The model under review builds one solid part; all positions refer to its coordinate system, in mm. A direction names the side the tool comes from. Round coordinates to 2 decimals unless told otherwise and drop trailing zeros. Order: outer loops, then holes, each group sorted by start corner. A loop starts at its lowest first (then second) coordinate and runs counter-clockwise, first axis right, second up. Notation, with made-up numbers: M 81,87 L 94,87 A20 cw 94,111 Z; hole C 33.25,64.5 d9. An arc over 180 degrees is marked long. One line per item, written item: value. Start each with the question number.
Autodesk Inventor part; units mm, degrees
ref_plane "2_XY" through (0, 3.15, 0) normal (1, 0, 0) x (0, 0, -1)
ref_plane "2_YZ" through (0, 3.15, 0) normal (0, 0, -1) x (0, 1, 0)
ref_plane "2_ZX" through (0, 3.15, 0) normal (0, 1, 0) x (1, 0, 0)
sketch "Sketch_1" plane through (0, 0, 0) normal (0, 1, 0) x (-1, 0, 0)
  line L0 (0, 16) -> (-25, 16)
  line L1 (-25, 16) -> (-25, 3.15)
  line L2 (-25, 3.15) -> (-20, 3.15)
  line L3 (-20, 3.15) -> (-20, 3.65)
  line L4 (-20, 3.65) -> (-15, 3.65)
  line L5 (-15, 3.65) -> (-15, 3.15)
  line L6 (-15, 3.15) -> (-10, 3.15)
  line L7 (-10, 3.15) -> (-10, 3.65)
  line L8 (-10, 3.65) -> (-5, 3.65)
  line L9 (-5, 3.65) -> (-5, 3.15)
  line L10 (-5, 3.15) -> (0, 3.15)
  line L11 (0, 3.15) -> (0, 16)
extrude "Extrusion1" add sketch "Sketch_1" along normal blind 1.5
sketch "Sketch_2" plane through (0, 0, 0) normal (1, 0, 0) x (0, 1, 0)
  line L0 (1.5, 10.6667) -> (0, 10.6667)
  line L1 (0, 10.6667) -> (0, 0)
  arc A0 (0, 0) -> (3.15, 3.15) centre (3.15, 0) ccw
  line L2 (3.15, 3.15) -> (1.5, 3.15)
  line L3 (1.5, 3.15) -> (1.5, 10.6667)
  circle A1 centre (3.15, 0) radius 1.5
extrude "Extrusion2" add sketch "Sketch_2" along normal blind 5
sketch "Sketch_3" plane through (10, 0, 0) normal (1, 0, 0) x (0, 0, -1)
  line L0 (-10.6667, 1.5) -> (-10.6667, 0)
  line L1 (-10.6667, 0) -> (0, 0)
  arc A0 (0, 0) -> (-3.15, 3.15) centre (0, 3.15) ccw
  line L2 (-3.15, 3.15) -> (-3.15, 1.5)
  line L3 (-3.15, 1.5) -> (-10.6667, 1.5)
  circle A1 centre (0, 3.15) radius 1.5
extrude "Extrusion3" add sketch "Sketch_3" along normal blind 5
sketch "Sketch_4" plane through (20, 0, 0) normal (1, 0, 0) x (0, 0, -1)
  line L0 (-10.6667, 1.5) -> (-10.6667, 0)
  line L1 (-10.6667, 0) -> (0, 0)
  arc A0 (0, 0) -> (-3.15, 3.15) centre (0, 3.15) ccw
  line L2 (-3.15, 3.15) -> (-3.15, 1.5)
  line L3 (-3.15, 1.5) -> (-10.6667, 1.5)
  circle A1 centre (0, 3.15) radius 1.5
extrude "Extrusion4" add sketch "Sketch_4" along normal blind 5
sketch "Sketch5" plane through (0, 0, 0) normal (0, -1, 0) x (1, 0, 0)
  point P0 (6, 10)
hole "Hole1" at (6, 0, 10) direction (0, 1, 0) diameter 3.4 depth 2
sketch "Sketch6" plane through (0, 0, 0) normal (0, -1, 0) x (1, 0, 0)
  point P0 (19, 10)
hole "Hole2" at (19, 0, 10) direction (0, 1, 0) diameter 3.4 depth 2
ref_plane "2_XY" through (0, 3.15, 0) normal (1, 0, 0) x (0, 0, -1)
ref_plane "2_YZ" through (0, 3.15, 0) normal (0, 0, -1) x (0, 1, 0)
ref_plane "2_ZX" through (0, 3.15, 0) normal (0, 1, 0) x (1, 0, 0)
properties part number "2HHKS25" material "ステンレス鋼"
Item 1: Consider section A-A, the plane z = 10. Give the boundary of the cut face in (x, y), then the cut area to 3 significant figures.
Item 2: The part is to be moulded in two halves that separate along Z. For faces 4 (the flat face through (22, 2, 3.15)), 5 (the flat face through (10, 1.7, 1)), 6 (the cylindrical face through (2.46, 4.58, -0.45)), say which applies: pulls with the +Z half, pulls with the -Z half, needs draft (parallel to the pull), parting line crosses it, or undercut.
Item 3: Consider section C-C, the plane x = 12. Give the boundary of the cut face in (y, z).
Item 4: Machinability: for faces 1 (the flat face through (2, 2, 3.15)), 2 (the flat face through (5, 1.7, 1.1)), 3 (the cylindrical face through (17.567, 0.76, 9.086)), which of the approach directions +Z, -Z, +X, -X, +Y, -Y give a long, thin tool a straight path to every point of the face, cutting with its end or side? Answer none if there is none.
Item 5: Consider section D-D, the plane y = 3.5. Give the boundary of the cut face in (x, z), then the cut area to 3 significant figures.
Item 6: Consider section B-B, the plane x = 6. Give the boundary of the cut face in (y, z), then the cut area to 3 significant figures.
Item 7: Wall thickness on L1, parallel to X at y = 1, z = -0.75; L2, parallel to X at y = 0.85, z = 10; L3, parallel to Y at x = 12.15, z = 0: over which ranges is each line inside the solid? List them lowest first.
Item 8: Clearance check with flat-ended pins moving along their axes: P1, Ø1.8, axis at x = 21.5, y = 2.5, coming from the +Z side; P2, Ø1.6, axis at x = 16.5, y = 0.5, coming from the -Z side; P3, Ø2, axis at x = 18, z = 3.5, coming from the +Y side; P4, Ø2.5, axis at y = 3.15, z = 0, coming from the -X side. State where each tip first meets the part, or that it passes through.
Computed:
1. outline: M 0,0 L 4.3,0 L 4.3,1.5 L 0,1.5 Z; M 7.7,0 L 17.3,0 L 17.3,1.5 L 7.7,1.5 Z; M 20.7,0 L 25,0 L 25,1.5 L 20.7,1.5 Z
1. area: 27.3 mm^2
2. face 4: pulls with the +Z half
2. face 5: needs draft
2. face 6: undercut
3. outline: M 0,0 A3.15 ccw long 3.15,3.15 L 1.5,3.15 L 1.5,16 L 0,16 Z; hole C 3.15,0 d3
4. face 1: +Z, +X, -X, +Y
4. face 2: -Z, +Y, -Y
4. face 3: +Y, -Y
5. outline: M 0,-3.13 L 5,-3.13 L 5,-1.46 L 0,-1.46 Z; M 0,1.46 L 5,1.46 L 5,3.13 L 0,3.13 Z; M 10,-3.13 L 15,-3.13 L 15,-1.46 L 10,-1.46 Z; M 10,1.46 L 15,1.46 L 15,3.13 L 10,3.13 Z; M 20,-3.13 L 25,-3.13 L 25,-1.46 L 20,-1.46 Z; M 20,1.46 L 25,1.46 L 25,3.13 L 20,3.13 Z
5. area: 50.2 mm^2
6. outline: M 0,3.65 L 1.5,3.65 L 1.5,8.3 L 0,8.3 Z; M 0,11.7 L 1.5,11.7 L 1.5,16 L 0,16 Z
6. area: 13.4 mm^2
7. L1: x = 0 to 5, 10 to 15, 20 to 25
7. L2: x = 0 to 4.3, 7.7 to 17.3, 20.7 to 25
7. L3: y = 0 to 1.65, 4.65 to 6.3
8. P1: stops at z = 3.15
8. P2: stops at z = 3.65
8. P3: stops at y = 1.5
8. P4: passes through
